The listing builds one solid part. Answer for the finished solid, in the listing's coordinates (mm). Round coordinates to 2 decimals unless told otherwise and drop trailing zeros. Loops run counter-clockwise (first coordinate to the right, second up) from the corner with the lowest first, then second, coordinate; pieces in that order, holes last. Notation, with made-up numbers: (29.25, 67.25) - (55.25, 67.25) arc R16 ccw to (55.25, 98.25) - close; hole circle Ø9 at (-18, -36). An arc over 180 degrees is marked (long way). Write item = value, one per line. Start each with the question number.
1) Section B-B, the plane z = -64.5 is taken. Determine the outline of the cut face in (x, y).
2) Straight lines are drawn through the part: line 1 along Y through (x, z) = (-126, -60); line 2 along Z through (x, y) = (59, -4.5); line 3 along Y through (x, z) = (15, -71). For each, find the intervals that lie inside material, in ascending order.
3) Section A-A, the plane x = -8 is taken. Determine the outline of the cut face in (y, z), and give its area (3 significant figures).
4) Given pin 1 Ø1.3 at (x, z) = (-38.5, -59) entering from -Y; pin 2 Ø2 at (x, y) = (81.5, -4) entering from +Z, each flat-ended and moving along its own axis, determine where each tip first touches the part or whether it passes through.
5) Section C-C, the plane y = -3.5 is taken. Determine the outline of the cut face in (x, z).
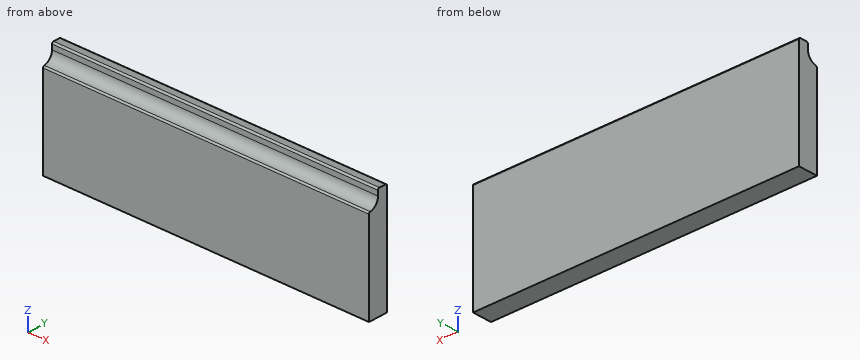
from build123d import *

# Parameters (mm, degrees)
F0_W     = 300
F0_H     = 100
F1_DEPTH = 9
F3_DEPTH = 300.001
F4_R     = 1.5


with BuildPart() as f1:
    # F0 (on Front) → F1 (new body, symmetric)
    with BuildSketch(Plane.XZ):
        with Locations((-3.7248600274, -105.7776198197)):
            Rectangle(F0_W, F0_H)
    extrude(amount=F1_DEPTH, both=True)

    # F2 (on face) → F3 (cut, through all)
    with BuildSketch(Plane.YZ.offset(146.2751399726)):
        with BuildLine():
            Line((0, -61.7776198197), (0, -55.7776198197))
            Line((0, -55.7776198197), (-9, -55.7776198197))
            Line((-9, -55.7776198197), (-9, -70.7776198197))
            ThreePointArc((-9, -70.7776198197), (-2.6360389693, -68.1415808503), (0, -61.7776198197))
        make_face()
    extrude(amount=-F3_DEPTH, mode=Mode.SUBTRACT)

    # F4
    f4_edges = [f1.edges().sort_by_distance(p)[0] for p in [
        (-3.72486, 0, -55.77762),
        (-3.72486, 9, -55.77762),
        (-3.72486, -9, -70.77762),
    ]]
    fillet(f4_edges, radius=F4_R)


solid = f1.part
Geometry check:
q1.outline = (-153.72, -0.42) - (146.28, -0.42) - (146.28, 9) - (-153.72, 9) - close
q2.line_1 = 0 to 9
q2.line_2 = -155.78 to -69.57
q2.line_3 = -8.44 to 9
q3.outline = (-9, -155.78) - (9, -155.78) - (9, -57.28) arc R1.5 ccw to (7.5, -55.78) - (1.5, -55.78) arc R1.5 ccw to (0, -57.28) - (0, -61.78) arc R9 cw to (-7.71, -70.69) arc R1.5 ccw to (-9, -72.17) - close
q3.area = 1,680 mm2
q4.pin_1 = 0
q4.pin_2 = -68.49
q5.outline = (-153.72, -155.78) - (146.28, -155.78) - (146.28, -68.9) - (-153.72, -68.9) - close
